Geometry check sheet. Reference: the model listing, model coordinates, mm. Face numbers are marked on the shaded views. A direction names the side the tool comes from. Give positions to 0.01 mm unless a question says otherwise; leave off trailing zeros. Write each loop counter-clockwise with the first axis right and the second up, starting at its lowest first coordinate (ties: lowest second). Pieces come first, ordered by that corner, then holes. Notation, with made-up numbers: M 75.5,28 L 131.5,28 A17 ccw 131.5,56 Z; hole C -22,-11.5 d1. An arc over 180 degrees is marked long. One line per item, written item: value. Start each with the question number.
1. Scan lines: line 1 (X direction, y = 2.3, z = -8.5); line 2 (X direction, y = 1.25, z = -18); line 3 (X direction, y = 2, z = -6.5). Record each from-to range of solid material in increasing order.
2. Cross-section at B-B on z = -8.5. Record the cut outline in (x, y), then the cut area to 3 significant figures.
3. Cross-section at A-A on y = 2. Record the cut outline in (x, z).
4. Release check for a two-part mould opening along X. For the marked faces 1, 2, 3 and 4 record: pulls with the +X half, pulls with the -X half, needs draft (parallel to the pull), parting line crosses it, or undercut.
5. Gauge pin test, flat ends, axial feed: pin 1 (3.5 mm diameter, centred on x = 10, z = -8.5, fed in from -Y); pin 2 (12.5 mm diameter, centred on x = 28, z = -16.5, fed in from +Y); pin 3 (8 mm diameter, centred on x = 9.5, z = -22, fed in from +Y). Record the tip position at first contact, or that the pin passes through.
6. Cross-section at D-D on x = 19.5. Record the cut outline in (y, z), then the cut area to 3 significant figures.
7. Tool access check on the marked faces 5, 6 and 7. Record the directions out of +Z, -Z, +X, -X, +Y, -Y that give a thin tool (end or side, any length) a straight path to the whole face; none if there is none.
8. Cross-section at C-C on x = 29. Record the cut outline in (y, z).
from build123d import *

# Parameters (mm, degrees)
CROQUIS1_W              = 39
CROQUIS1_H              = 31
CROQUIS1_R              = 2.25
SALIENTE_EXTRUIR1_DEPTH = 4
CROQUIS2_R              = 4
SALIENTE_EXTRUIR2_DEPTH = 31
CROQUIS3_W              = 1.5
CROQUIS3_H              = 4
CORTAR_EXTRUIR1_DEPTH   = 31
REDONDEO1_R             = 2


with BuildPart() as part:
    # Croquis1 → Saliente-Extruir1 (new body)
    with BuildSketch(Plane(origin=(0, 0, 0), x_dir=(1, 0, 0), z_dir=(0, 1, 0))):
        with Locations((19.5, 15.5)):
            Rectangle(CROQUIS1_W, CROQUIS1_H)
        with Locations(Location((10, 22.5, 0), (0, 0, 270))):
            Circle(CROQUIS1_R, mode=Mode.SUBTRACT)
        with Locations(Location((29, 22.5, 0), (0, 0, 270))):
            Circle(CROQUIS1_R, mode=Mode.SUBTRACT)
        with Locations(Location((29, 8.5, 0), (0, 0, 270))):
            Circle(CROQUIS1_R, mode=Mode.SUBTRACT)
        with Locations(Location((10, 8.5, 0), (0, 0, 270))):
            Circle(CROQUIS1_R, mode=Mode.SUBTRACT)
    extrude(amount=SALIENTE_EXTRUIR1_DEPTH)

    # Croquis2 → Saliente-Extruir2 (add)
    with BuildSketch(Plane.XY):
        with Locations((19.5, 4)):
            Circle(CROQUIS2_R)
    extrude(amount=-SALIENTE_EXTRUIR2_DEPTH)

    # Croquis3 → Cortar-Extruir1 (cut)
    with BuildSketch(Plane(origin=(0, 0, -31), x_dir=(-1, 0, 0), z_dir=(0, 0, -1))):
        with Locations((-19.5, 2)):
            Rectangle(CROQUIS3_W, CROQUIS3_H)
    extrude(amount=-CORTAR_EXTRUIR1_DEPTH, mode=Mode.SUBTRACT)

    # Redondeo1
    redondeo1_edges = [part.edges().sort_by_distance(p)[0] for p in [
        (0, 2, -31),
        (39, 2, -31),
        (39, 2, 0),
        (0, 2, 0),
    ]]
    fillet(redondeo1_edges, radius=REDONDEO1_R)


solid = part.part
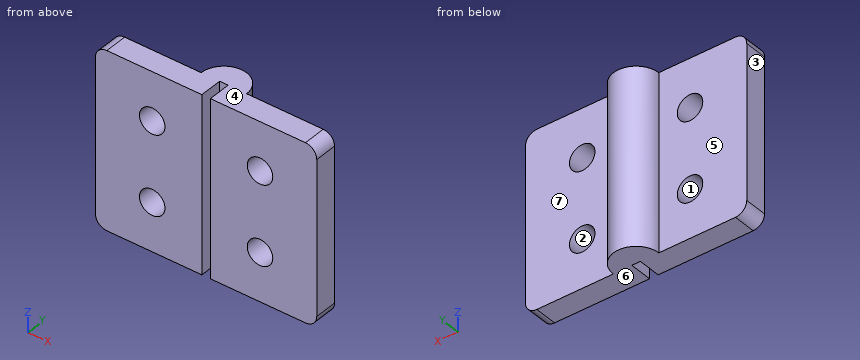
Report:
1. line 1: x = 0 to 7.75, 12.25 to 18.75, 20.25 to 26.75, 31.25 to 39
1. line 2: x = 0 to 18.75, 20.25 to 39
1. line 3: x = 0 to 8.97, 11.03 to 18.75, 20.25 to 27.97, 30.03 to 39
2. outline: M 0,0 L 7.75,0 L 7.75,4 L 0,4 Z; M 12.25,0 L 18.75,0 L 18.75,4 L 20.25,4 L 20.25,0 L 26.75,0 L 26.75,4 L 23.5,4 A4 ccw 15.5,4 L 12.25,4 Z; M 31.25,0 L 39,0 L 39,4 L 31.25,4 Z
2. area: 139 mm^2
3. outline: M 0,-29 A2 ccw 2,-31 L 18.75,-31 L 18.75,0 L 2,0 A2 ccw 0,-2 Z; M 20.25,-31 L 37,-31 A2 ccw 39,-29 L 39,-2 A2 ccw 37,0 L 20.25,0 Z; hole C 10,-22.5 d4.5; hole C 10,-8.5 d4.5; hole C 29,-22.5 d4.5; hole C 29,-8.5 d4.5
4. face 1: undercut
4. face 2: undercut
4. face 3: pulls with the -X half
4. face 4: needs draft
5. pin 1: passes through
5. pin 2: stops at y = 7.31
5. pin 3: stops at y = 4
6. outline: M 4,-31 L 8,-31 L 8,0 L 4,0 Z
6. area: 124 mm^2
7. face 5: +Z, -Z, -X, +Y
7. face 6: -Z, +X, -X, +Y, -Y
7. face 7: +Z, -Z, +X, +Y
8. outline: M 0,-31 L 4,-31 L 4,-24.75 L 0,-24.75 Z; M 0,-20.25 L 4,-20.25 L 4,-10.75 L 0,-10.75 Z; M 0,-6.25 L 4,-6.25 L 4,0 L 0,0 Z
